Verification items for the finished model (mm, model axes). Face numbers are marked on the shaded views. A direction names the side the tool comes from. Round coordinates to 2 decimals unless told otherwise and drop trailing zeros. Order: outer loops, then holes, each group sorted by start corner. A loop starts at its lowest first (then second) coordinate and runs counter-clockwise, first axis right, second up. Notation, with made-up numbers: M 51.5,47.25 L 89.5,47.25 A20 ccw 89.5,57.25 Z; hole C 15,87.5 d5. An arc over 180 degrees is marked long. Use CSV: the item, a comma, the result in double quotes. Start each with the question number.
Q1. Sectioned sample at C-C (y = 63.5). Enter the section's corners in (x, z), and give its area (3 significant figures).
Q2. Scan lines: line 1 (Z direction, x = 8, y = 68); line 2 (Y direction, x = 15.5, z = 18.25); line 3 (Y direction, x = 2, z = 9.25). Record each from-to range of solid material in increasing order.
Q3. Sectioned sample at D-D (x = 59.5). Enter the section's corners in (y, z).
Q4. Set-up check for the marked faces 1 and 2: record each of +Z, -Z, +X, -X, +Y, -Y from which the full face is reachable in a straight line by a thin tool's end or side.
Q5. Gauge pin test, flat ends, axial feed: pin 1 Ø1.7 at (x, z) = (-8, 9.5) entering from -Y; pin 2 Ø6 at (x, y) = (5, 72) entering from -Z; pin 3 Ø6 at (x, z) = (46, 16) entering from -Y; pin 4 Ø5 at (y, z) = (96.5, 9.5) entering from -X. Record the tip position at first contact, or that the pin passes through.
Q6. Sectioned sample at B-B (z = 21.75). Enter the section's corners in (x, y), and give its area (3 significant figures).
Q7. Sectioned sample at A-A (z = 12.5). Enter the section's corners in (x, y), and give its area (3 significant figures).
```python
from build123d import *

# Parameters (mm, degrees)
SKETCH_1_W          = 26.239617318
SKETCH_1_H          = 120
EXTRUDE_1_DEPTH     = 25
CHAMFER_1_SIZE      = 8
SKETCH_3_W          = 15
SKETCH_3_H          = 15
CUT_EXTRUDE_4_DEPTH = 35
SKETCH_4_R          = 5
EXTRUDE_2_DEPTH     = 15
SKETCH_5_R          = 10.513466809
SKETCH_5_R_2        = 5
CUT_EXTRUDE_5_DEPTH = 15
SKETCH_6_W          = 15
SKETCH_6_H          = 15
CUT_EXTRUDE_6_DEPTH = 188.870930903
SKETCH_7_R          = 5
EXTRUDE_3_DEPTH     = 15
SKETCH_8_R          = 5
CUT_EXTRUDE_9_DEPTH = 15


with BuildPart() as part:
    # 草图1 → 凸台-拉伸1 (new body)
    with BuildSketch(Plane.XY):
        with Locations((3.568688241, 27.453328425)):
            Rectangle(SKETCH_1_W, SKETCH_1_H)
        Polygon((52.421783721, 135.65221029), (16.6884969, 87.453328425), (-9.551120418, 87.453328425), (33.944293966, 140.364941184), (82.783975756, 161.693279677), align=None)
    extrude(amount=EXTRUDE_1_DEPTH)

    # 倒角1
    chamfer_1_edges = [part.edges().sort_by_distance(p)[0] for p in [
        (16.6884969, -32.546671575, 12.5),
        (-9.551120418, -32.546671575, 12.5),
    ]]
    chamfer(chamfer_1_edges, length=CHAMFER_1_SIZE)

    # 草图3 → 切除-拉伸4 (cut)
    with BuildSketch(Plane.ZY.offset(9.551120418)):
        with Locations((12.5, -12.627226007)):
            Rectangle(SKETCH_3_W, SKETCH_3_H)
    extrude(amount=-CUT_EXTRUDE_4_DEPTH, mode=Mode.SUBTRACT)

    # 草图4 → 凸台-拉伸2 (add)
    with BuildSketch(Plane.XY.offset(5)):
        with Locations(Location((3.568688241, -12.627226007, 0), (0, 0, 180))):
            Circle(SKETCH_4_R)
    extrude(amount=EXTRUDE_2_DEPTH)

    # 草图5 → 切除-拉伸5 (cut)
    with BuildSketch(Plane.XY.offset(5)):
        with Locations((3.568688241, -12.627226007)):
            Circle(SKETCH_5_R)
        with Locations(Location((3.568688241, -12.627226007, 0), (0, 0, 180))):
            Circle(SKETCH_5_R_2, mode=Mode.SUBTRACT)
    extrude(amount=CUT_EXTRUDE_5_DEPTH, mode=Mode.SUBTRACT)

    # 草图6 → 切除-拉伸6 (cut, through all)
    with BuildSketch(Plane.ZY.offset(9.551120418)):
        with Locations((12.5, 75.533882858)):
            Rectangle(SKETCH_6_W, SKETCH_6_H)
    extrude(amount=-CUT_EXTRUDE_6_DEPTH, mode=Mode.SUBTRACT)

    # 草图7 → 凸台-拉伸3 (add)
    with BuildSketch(Plane.XY.offset(5)):
        with Locations(Location((3.568688241, 75.533882858, 0), (0, 0, 180))):
            Circle(SKETCH_7_R)
    extrude(amount=EXTRUDE_3_DEPTH)

    # 草图8 → 切除-拉伸9 (cut)
    # profile 1 of 3: a face of its own
    with BuildSketch(Plane.XY.offset(5)):
        with BuildLine():
            ThreePointArc((13.459511585, 75.533882858), (12.557728949, 79.660083722), (10.016818701, 83.033882858))
            Line((10.016818701, 83.033882858), (-2.879442218, 83.033882858))
            ThreePointArc((-2.879442218, 83.033882858), (-6.322135103, 75.533882858), (-2.879442218, 68.033882858))
            Line((-2.879442218, 68.033882858), (10.016818701, 68.033882858))
            ThreePointArc((10.016818701, 68.033882858), (12.557728949, 71.407681993), (13.459511585, 75.533882858))
        make_face()
        with Locations(Location((3.568688241, 75.533882858, 0), (0, 0, 180))):
            Circle(SKETCH_8_R, mode=Mode.SUBTRACT)
    # profile 2 of 3: a face of its own
    with BuildSketch(Plane.XY.offset(5)):
        with BuildLine():
            Line((-2.879442218, 83.033882858), (10.016818701, 83.033882858))
            ThreePointArc((10.016818701, 83.033882858), (3.568688241, 85.424706202), (-2.879442218, 83.033882858))
        make_face()
    # profile 3 of 3: a face of its own
    with BuildSketch(Plane.XY.offset(5)):
        with BuildLine():
            ThreePointArc((-2.879442218, 68.033882858), (3.568688241, 65.643059514), (10.016818701, 68.033882858))
            Line((10.016818701, 68.033882858), (-2.879442218, 68.033882858))
        make_face()
    extrude(amount=CUT_EXTRUDE_9_DEPTH, mode=Mode.SUBTRACT)


solid = part.part
```
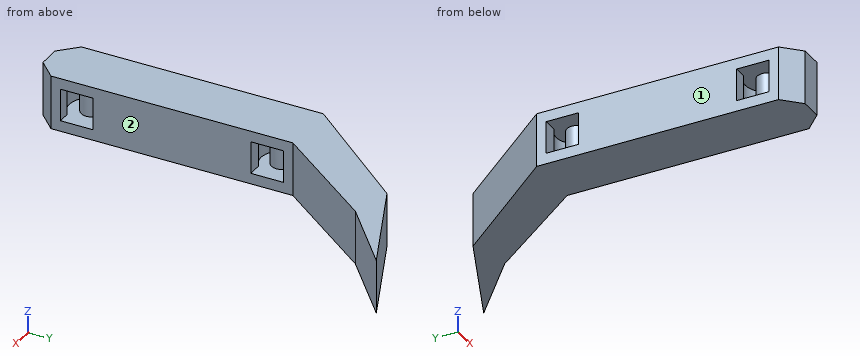
Verdict:
1,outline,"M -9.55,0 L 16.69,0 L 16.69,25 L -9.55,25 Z"
1,area,"656 mm²"
2,line 1,"z = 0 to 5, 20 to 25"
2,line 2,"y = -25.74 to -20.13, -5.13 to 68.03, 83.03 to 117.93"
2,line 3,"y = -32.55 to -23.02, -17.37 to -7.88, -2.23 to 65.77, 70.79 to 80.28, 85.3 to 101.51"
3,outline,"M 141.72,0 L 151.53,0 L 151.53,25 L 141.72,25 Z"
4,face 1,"+Z, -Z, -X, +Y, -Y"
4,face 2,"+Z, -Z, +X, -Y"
5,pin 1,"stops at y = -26.95"
5,pin 2,"stops at z = 0"
5,pin 3,"stops at y = 122.94"
5,pin 4,"stops at x = -4.17"
6,outline,"M -9.55,-24.55 L -1.55,-32.55 L 8.69,-32.55 L 16.69,-24.55 L 16.69,87.45 L 52.42,135.65 L 82.78,161.69 L 33.94,140.36 L -9.55,87.45 Z"
6,area,"4,620 mm²"
7,outline,"M -9.55,-24.55 L -1.55,-32.55 L 8.69,-32.55 L 16.69,-24.55 L 16.69,-20.13 L 10.94,-20.13 A10.51 cw -3.8,-20.13 L -9.55,-20.13 Z; M -9.55,-5.13 L -3.8,-5.13 A10.51 cw 10.94,-5.13 L 16.69,-5.13 L 16.69,68.03 L 10.02,68.03 A9.89 cw -2.88,68.03 L -9.55,68.03 Z; M -9.55,83.03 L -2.88,83.03 A9.89 cw 10.02,83.03 L 16.69,83.03 L 16.69,87.45 L 52.42,135.65 L 82.78,161.69 L 33.94,140.36 L -9.55,87.45 Z; C 3.57,-12.63 d10; C 3.57,75.53 d10"
7,area,"3,890 mm²"
